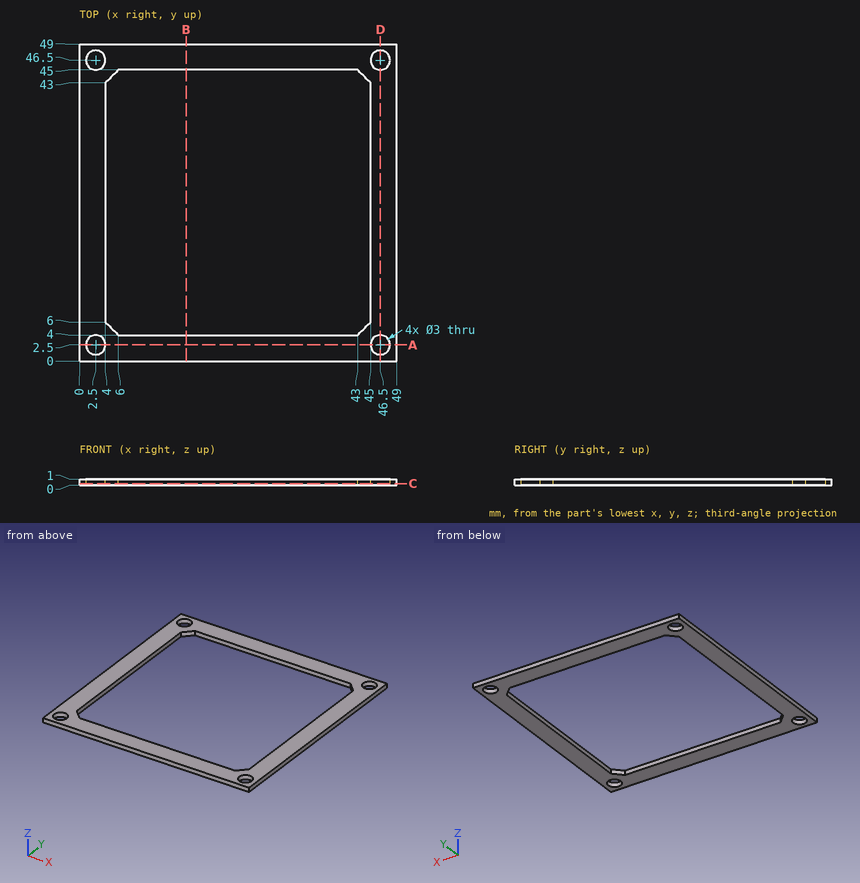
Design review of the part shown in the three views and the two pictorial views. Dimensions are in mm from the part's minimum x, y and z. Round coordinates to 2 decimals unless told otherwise and drop trailing zeros. Loops run counter-clockwise (first coordinate to the right, second up) from the corner with the lowest first, then second, coordinate; pieces in that order, holes last. Notation, with made-up numbers: M 41,43 L 95,43 A20 cw 95,78 Z; hole C 49.25,7.25 d1. An arc over 180 degrees is marked long. Answer as a JSON object with one key per item and string values.
Item 1: Clearance check with flat-ended pins moving along their axes: P1, Ø2.5, axis at x = 46.5, y = 46.5, coming from the +Z side; P2, Ø4, axis at x = 2.5, y = 46.5, coming from the +Z side. State where each tip first meets the part, or that it passes through.
Answer sheet:
{"P1": "passes through", "P2": "stops at z = 1"}
Item 2: Wall thickness on L1, parallel to X at y = 2.5, z = 0.3; L2, parallel to Y at x = 35.5, z = 0.5: over which ranges is each line inside the solid? List them lowest first. Write a range as from..to.
Answer sheet:
{"L1": "x = 0..1, 4..45, 48..49", "L2": "y = 0..4, 45..49"}
Item 3: We need section B-B on x = 16.5. Give the boundary of the cut face in (y, z), and give its area (3 significant figures).
Answer sheet:
{"outline": "M 0,0 L 4,0 L 4,1 L 0,1 Z; M 45,0 L 49,0 L 49,1 L 45,1 Z", "area": "8.00 mm^2"}
Item 4: We need section C-C on z = 0.3. Give the boundary of the cut face in (x, y).
Answer sheet:
{"outline": "M 0,0 L 49,0 L 49,49 L 0,49 Z; hole C 2.5,2.5 d3; hole C 2.5,46.5 d3; hole M 4,6 L 6,4 L 43,4 L 45,6 L 45,43 L 43,45 L 6,45 L 4,43 Z; hole C 46.5,2.5 d3; hole C 46.5,46.5 d3"}
Item 5: We need section A-A on y = 2.5. Give the boundary of the cut face in (x, z).
Answer sheet:
{"outline": "M 0,0 L 1,0 L 1,1 L 0,1 Z; M 4,0 L 45,0 L 45,1 L 4,1 Z; M 48,0 L 49,0 L 49,1 L 48,1 Z"}
